```python
from build123d import *

# Parameters (mm, degrees)
BOSS_EXTRUDE3_DEPTH     = 6
SHELL2_T                = -2
CUT_EXTRUDE4_DEPTH      = 32
CUT_EXTRUDE4_DEPTH_BACK = 34.275216002
SKETCH2_R               = 1.5
SKETCH2_R_2             = 1.407616296
SKETCH2_R_3             = 1.41
SKETCH2_W               = 1.407616296
SKETCH2_H               = 2.445621179
SKETCH2_W_2             = 1.376750608
SKETCH7_R               = 2.502744699
SKETCH7_R_2             = 1.5
BOSS_EXTRUDE4_DEPTH     = 6
SKETCH8_R               = 2.53531283
SKETCH8_R_2             = 1.518842354
BOSS_EXTRUDE6_DEPTH     = 4
FILLET1_R               = 2
FILLET2_R               = 2
CUT_EXTRUDE6_REACH      = 40.307
SKETCH10_W              = 14.351477832
SKETCH10_H              = 5
FILLET3_R               = 1
SKETCH11_R              = 3.20834654
SKETCH11_R_2            = 3.35149953
CUT_EXTRUDE7_DEPTH      = 0.4
SKETCH14_W              = 23
SKETCH14_H              = 23.8
BOSS_EXTRUDE9_DEPTH     = 2
BOSS_EXTRUDE10_DEPTH    = 2
SKETCH16_R              = 1.5
SKETCH16_R_2            = 1.407616296
SKETCH16_R_3            = 1.41
SKETCH16_W              = 2.806264375
SKETCH16_H              = 2.502132393
SKETCH16_W_2            = 2.82
SKETCH16_H_2            = 2.45355852
CUT_EXTRUDE9_DEPTH      = 33.299225997
SKETCH17_R              = 3.066424979
SKETCH17_R_2            = 3.059739342
CUT_EXTRUDE10_DEPTH     = 1


with BuildPart() as part:
    # Sketch1 → Boss-Extrude3 (new body)
    with BuildSketch(Plane(origin=(0, 0, 0), x_dir=(1, 0, 0), z_dir=(0, 1, 0))):
        Polygon((0, -7), (-17, -7), (-17, 17.8), (-17, 26.8), (16, 26.8), (16, 17.8), (16, -7), align=None)
    extrude(amount=BOSS_EXTRUDE3_DEPTH)

    # Shell2
    shell2_openings = [part.faces().sort_by_distance(p)[0] for p in [
        (-0.5, 0, -9.9),
    ]]
    offset(amount=SHELL2_T, openings=shell2_openings, kind=Kind.INTERSECTION)

    # Sketch2 → Cut-Extrude4 (cut, two sides: drawn at the far end of the back side and taken through both)
    with BuildSketch(Plane(origin=(0, 10, 0), x_dir=(1, 0, 0), z_dir=(0, 1, 0)).offset(-CUT_EXTRUDE4_DEPTH_BACK)):
        with Locations(Location((0, 17.8, 0), (0, 0, 270))):
            Circle(SKETCH2_R)
        with Locations((-8.22, 9.5)):
            Circle(SKETCH2_R_2)
        with Locations((7.58, 9.5)):
            Circle(SKETCH2_R_3)
        with Locations(Location((0, 0, 0), (0, 0, 270))):
            Circle(SKETCH2_R)
        with Locations((-7.516191852, 8.277189411)):
            Rectangle(SKETCH2_W, SKETCH2_H)
        with Locations((6.891624696, 8.277189411)):
            Rectangle(SKETCH2_W_2, SKETCH2_H)
    extrude(amount=CUT_EXTRUDE4_DEPTH + CUT_EXTRUDE4_DEPTH_BACK, mode=Mode.SUBTRACT)

    # Sketch7 → Boss-Extrude4 (add)
    with BuildSketch(Plane(origin=(0, 6, 0), x_dir=(1, 0, 0), z_dir=(0, 1, 0))):
        with Locations(Location((0, 17.8, 0), (0, 0, 270))):
            Circle(SKETCH7_R)
        with Locations(Location((0, 17.8, 0), (0, 0, 270))):
            Circle(SKETCH7_R_2, mode=Mode.SUBTRACT)
    extrude(amount=-BOSS_EXTRUDE4_DEPTH)

    # Sketch8 → Boss-Extrude6 (add)
    with BuildSketch(Plane.XZ.offset(-4)):
        with Locations(Location((0, 0, 0), (0, 0, 90))):
            Circle(SKETCH8_R)
        with Locations(Location((0, 0, 0), (0, 0, 90))):
            Circle(SKETCH8_R_2, mode=Mode.SUBTRACT)
    extrude(amount=BOSS_EXTRUDE6_DEPTH)

    # Fillet1
    fillet1_edges = [part.edges().sort_by_distance(p)[0] for p in [
        (-17, 3, 7),
        (-17, 3, -26.8),
        (16, 3, -26.8),
        (16, 3, 7),
    ]]
    fillet(fillet1_edges, radius=FILLET1_R)

    # Fillet2
    fillet2_edges = [part.edges().sort_by_distance(p)[0] for p in [
        (14, 2, 5),
        (14, 2, -24.8),
        (-15, 2, -24.8),
        (-15, 2, 5),
    ]]
    fillet(fillet2_edges, radius=FILLET2_R)

    # Sketch10 → Cut-Extrude6 (cut, up to next)
    with BuildSketch(Plane.XY.offset(7), mode=Mode.PRIVATE) as cut_extrude6_sk1:
        with Locations((0.071944839, 0.064631552)):
            Rectangle(SKETCH10_W, SKETCH10_H)
    cut_extrude6_tool1 = extrude(cut_extrude6_sk1.sketch, amount=-CUT_EXTRUDE6_REACH, mode=Mode.PRIVATE) & part.part
    add(cut_extrude6_tool1.solids().sort_by_distance((0.071945, 0.064632, 7))[0], mode=Mode.SUBTRACT)

    # Fillet3
    fillet3_edges = [part.edges().sort_by_distance(p)[0] for p in [
        (7.247683755, 2.564631552, 6),
        (-7.103794077, 2.564631552, 6),
    ]]
    fillet(fillet3_edges, radius=FILLET3_R)

    # Sketch11 → Cut-Extrude7 (cut)
    with BuildSketch(Plane.XZ):
        Circle(SKETCH11_R)
        with Locations((0, -17.8)):
            Circle(SKETCH11_R_2)
    extrude(amount=-CUT_EXTRUDE7_DEPTH, mode=Mode.SUBTRACT)

    # Sketch14 → Boss-Extrude9 (add)
    with BuildSketch(Plane(origin=(0, 6, 0), x_dir=(1, 0, 0), z_dir=(0, 1, 0))):
        with Locations((-0.5, 9.9)):
            Rectangle(SKETCH14_W, SKETCH14_H)
    extrude(amount=BOSS_EXTRUDE9_DEPTH)

    # Sketch15 → Boss-Extrude10 (add)
    with BuildSketch(Plane(origin=(0, 8, 0), x_dir=(1, 0, 0), z_dir=(0, 1, 0))):
        with BuildLine():
            Line((14, -3), (14, 22.8))
            ThreePointArc((14, 22.8), (13.414213562, 24.214213562), (12, 24.8))
            Line((12, 24.8), (-13, 24.8))
            ThreePointArc((-13, 24.8), (-14.414213562, 24.214213562), (-15, 22.8))
            Line((-15, 22.8), (-15, -3))
            ThreePointArc((-15, -3), (-14.414213562, -4.414213562), (-13, -5))
            Line((-13, -5), (12, -5))
            ThreePointArc((12, -5), (13.414213562, -4.414213562), (14, -3))
        make_face()
    extrude(amount=BOSS_EXTRUDE10_DEPTH)

    # Sketch16 → Cut-Extrude9 (cut, through all)
    with BuildSketch(Plane.XZ.offset(-4)):
        with Locations(Location((0, 0, 0), (0, 0, 270))):
            Circle(SKETCH16_R)
        with Locations(Location((0, -17.8, 0), (0, 0, 270))):
            Circle(SKETCH16_R)
        with Locations((-8.22, -9.5)):
            Circle(SKETCH16_R_2)
        with Locations((7.58, -9.5)):
            Circle(SKETCH16_R_3)
        with Locations((-8.215515892, -8.248933803)):
            Rectangle(SKETCH16_W, SKETCH16_H)
        with Locations((7.58, -8.27322074)):
            Rectangle(SKETCH16_W_2, SKETCH16_H_2)
    extrude(amount=-CUT_EXTRUDE9_DEPTH, mode=Mode.SUBTRACT)

    # Sketch17 → Cut-Extrude10 (cut)
    with BuildSketch(Plane(origin=(0, 10, 0), x_dir=(1, 0, 0), z_dir=(0, 1, 0))):
        with Locations(Location((0, 17.8, 0), (0, 0, 270))):
            Circle(SKETCH17_R)
        with Locations(Location((0, 0, 0), (0, 0, 270))):
            Circle(SKETCH17_R_2)
    extrude(amount=-CUT_EXTRUDE10_DEPTH, mode=Mode.SUBTRACT)


solid = part.part
```
Work out the finished part from the listing and answer in its coordinate system (mm). A direction names the side the tool comes from. Give positions to 0.01 mm unless a question says otherwise; leave off trailing zeros. Loops run counter-clockwise (first coordinate to the right, second up) from the corner with the lowest first, then second, coordinate; pieces in that order, holes last. Notation, with made-up numbers: (-5, 49.5) - (49, 49.5) arc R17 ccw to (49, 57.5) - close; hole circle Ø8 at (89.5, -2.75). An arc over 180 degrees is marked (long way). Use CSV: the item, a comma, the result in double quotes. Start each with the question number.
(1) Determine the mould class of faces 1 (the face through (-1, 9, 5)), 2 (the face through (1, 9, -16)), 3 (the face through (-17, 3, -10)) for opening direction Z: released by +Z, released by -Z, zero draft, split by the parting line, or undercut.
(2) A tool of negligible diameter and unlimited length cuts with its end or side. For faces 4 (the face through (-15, 2, -10)), 5 (the face through (14, 9, -10)), 6 (the face through (7.248, 1, 6)), from which of +Z, -Z, +X, -X, +Y, -Y can it reach the whole face along a straight path? Write none if from no direction.
(3) Find the intervals of material crossed by L1, parallel to Z at x = 0, y = 6.75; L2, parallel to X at y = 2, z = -17.8; L3, parallel to Z at x = -11, y = 2.5, in increasing order.
(4) Find section C-C, the plane y = 4.5. Determine the outline of the cut face in (x, z), plus the area to 3 significant figures.
(5) Find section D-D, the plane z = -24. Determine the outline of the cut face in (x, y), plus the area to 3 significant figures.
(6) Find section B-B, the plane x = -8.22. Determine the outline of the cut face in (y, z).
(7) Each of these flat-tipped pins is pushed along its axis until it touches: pin 1 (2 mm diameter, centred on y = 9, z = -7.5, fed in from +X); pin 2 (1 mm diameter, centred on x = 2, z = 6.5, fed in from -Y); pin 3 (4 mm diameter, centred on x = 1.5, z = 2.5, fed in from +Y); pin 4 (0.7 mm diameter, centred on y = 8, z = -8, fed in from -X). Where does it stop, or does it pass through?
Results found:
1,face 1,"released by +Z"
1,face 2,"undercut"
1,face 3,"zero draft"
2,face 4,"-Y"
2,face 5,"+Z, -Z, +X, +Y"
2,face 6,"+Z, -Y"
3,L1,"-21.8 to -19.3, -16.3 to -1.5, 1.5 to 2"
3,L2,"-17 to -15, -2.5 to -1.5, 1.5 to 2.5, 14 to 16"
3,L3,"-26.8 to -24.8, 5 to 7"
4,outline,"(-17, -24.8) arc R2 ccw to (-15, -26.8) - (14, -26.8) arc R2 ccw to (16, -24.8) - (16, 5) arc R2 ccw to (14, 7) - (-15, 7) arc R2 ccw to (-17, 5) - close; hole (-9.62, -9.34) arc R1.41 ccw (long way) to (-6.81, -9.5) - (-6.81, -7) - (-9.62, -7) - close; hole circle Ø3 at (0, -17.8); hole circle Ø3 at (0, 0); hole (6.17, -9.5) arc R1.41 ccw to (8.99, -9.5) - (8.99, -7.05) - (6.17, -7.05) - close"
4,area,"1,080 mm^2"
5,outline,"(-17, 0) - (-14.6, 0) - (-14.6, 4) - (13.6, 4) - (13.6, 0) - (16, 0) - (16, 6) - (-17, 6) - close; (-14.6, 8) - (13.6, 8) - (13.6, 10) - (-14.6, 10) - close"
5,area,"142 mm^2"
6,outline,"(0, -26.8) - (6, -26.8) - (6, -21.8) - (8, -21.8) - (8, -24.8) - (10, -24.8) - (10, -10.91) - (4, -10.91) - (4, -24.8) - (0, -24.8) - close; (0, 5) - (4, 5) - (4, -7) - (10, -7) - (10, 5) - (8, 5) - (8, 2) - (6, 2) - (6, 7) - (0, 7) - close"
7,pin 1,"x = 14"
7,pin 2,"y = 2.56"
7,pin 3,"y = 10"
7,pin 4,"x = -15"
